Geometry check sheet. Reference: the model listing, model coordinates, mm. Face numbers are marked on the shaded views. A direction names the side the tool comes from. Coordinates: 2 decimals unless noted, no trailing zeros. Loops run counter-clockwise (first coordinate to the right, second up) from the corner with the lowest first, then second, coordinate; pieces in that order, holes last. Notation, with made-up numbers: M 88.5,74 L 118.5,74 A16 cw 118.5,90 Z; hole C -12.75,27 d6. An arc over 180 degrees is marked long. Use CSV: the item, a comma, the result in double quotes.
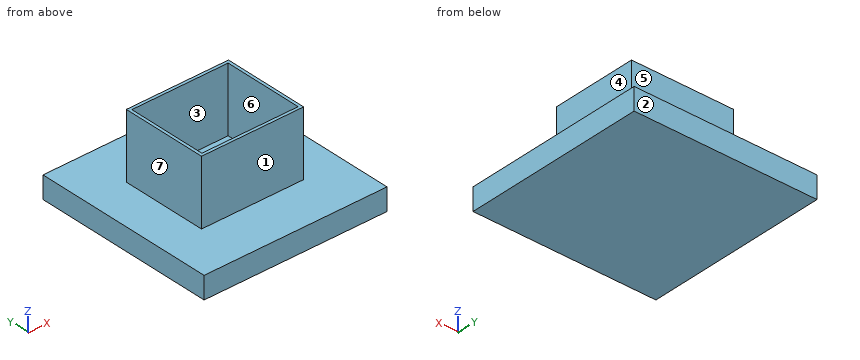
Autodesk Inventor part; units mm, degrees
ref_plane "YZ Plane" through (0, 0, 0) normal (1, 0, 0) x (0, 1, 0)
ref_plane "XZ Plane" through (0, 0, 0) normal (0, 1, 0) x (-1, 0, 0)
ref_plane "XY Plane" through (0, 0, 0) normal (0, 0, 1) x (1, 0, 0)
sketch "Sketch1" plane through (0, 0, 0) normal (0, 0, 1) x (1, 0, 0)
  line L0 (-17.15, -17.15) -> (17.15, -17.15)
  line L1 (17.15, -17.15) -> (17.15, 17.15)
  line L2 (17.15, 17.15) -> (-17.15, 17.15)
  line L3 (-17.15, 17.15) -> (-17.15, -17.15)
  line L4 (-17.15, -17.15) -> (17.15, 17.15) construction
  line L5 (17.15, -17.15) -> (-17.15, 17.15) construction
  point P0 (0, 0)
  dimension "d0" = 34.3
  dimension "d1" = 34.3
extrude "Extrusion1" add sketch "Sketch1" along normal blind 4.15
sketch "Sketch2" plane through (0, 0, 4.15) normal (0, 0, 1) x (1, 0, 0)
  line L0 (-9.025, -7.45) -> (9.025, -7.45)
  line L1 (9.025, -7.45) -> (9.025, 7.45)
  line L2 (9.025, 7.45) -> (-9.025, 7.45)
  line L3 (-9.025, 7.45) -> (-9.025, -7.45)
  line L4 (-9.025, -7.45) -> (9.025, 7.45) construction
  line L5 (9.025, -7.45) -> (-9.025, 7.45) construction
  line L6 (-9.5751, 8.0001) -> (9.5751, 8.0001)
  line L7 (9.5751, 8.0001) -> (9.5751, -8.0001)
  line L8 (9.5751, -8.0001) -> (-9.5751, -8.0001)
  line L9 (-9.5751, -8.0001) -> (-9.5751, 8.0001)
  point P0 (0, 0)
  dimension "d4" = 18.05
  dimension "d5" = 14.9
extrude "Extrusion2" add sketch "Sketch2" along normal blind 12.25
properties part number "RJ45_bulkhead"
1. Section check C-C, the plane x = 3. Record the cut outline in (y, z).
The answers:
outline,"M -17.15,0 L 17.15,0 L 17.15,4.15 L 8,4.15 L 8,16.4 L 7.45,16.4 L 7.45,4.15 L -7.45,4.15 L -7.45,16.4 L -8,16.4 L -8,4.15 L -17.15,4.15 Z"
2. Section check A-A, the plane z = 13.5. Record the cut outline in (x, y) (3 decimals).
The answers:
outline,"M -9.575,-8 L 9.575,-8 L 9.575,8 L -9.575,8 Z; hole M -9.025,-7.45 L 9.025,-7.45 L 9.025,7.45 L -9.025,7.45 Z"
3. Section check B-B, the plane y = -3.5. Record the cut outline in (x, z) (3 decimals), plus the area to 3 significant figures.
The answers:
outline,"M -17.15,0 L 17.15,0 L 17.15,4.15 L 9.575,4.15 L 9.575,16.4 L 9.025,16.4 L 9.025,4.15 L -9.025,4.15 L -9.025,16.4 L -9.575,16.4 L -9.575,4.15 L -17.15,4.15 Z"
area,"156 mm^2"
4. Gauge pin test, flat ends, axial feed: P1, Ø3.5, axis at x = -3, z = 9, coming from the +Y side; P2, Ø3.5, axis at y = -2.5, z = 11, coming from the +X side; P3, Ø1.5, axis at y = 5.5, z = 5, coming from the -X side. Record the tip position at first contact, or that the pin passes through.
The answers:
P1,"y = 8"
P2,"x = 9.58"
P3,"x = -9.58"
5. Section check D-D, the plane y = 14. Record the cut outline in (x, z), plus the area to 3 significant figures.
The answers:
outline,"M -17.15,0 L 17.15,0 L 17.15,4.15 L -17.15,4.15 Z"
area,"142 mm^2"
6. Thickness scan on line 1 (X direction, y = -3, z = 12) (3 decimals); line 2 (Y direction, x = -2, z = 13); line 3 (Z direction, x = -4, y = 14.5). Record the ranges inside material, lowest first. Write a range as [from, to].
The answers:
line 1,"[-9.575, -9.025], [9.025, 9.575]"
line 2,"[-8, -7.45], [7.45, 8]"
line 3,"[0, 4.15]"
7. Set-up check for the marked faces 1, 2 and 3: record each of +Z, -Z, +X, -X, +Y, -Y from which the full face is reachable in a straight line by a thin tool's end or side.
The answers:
face 1,"+Z, +X, -X, -Y"
face 2,"+Z, -Z, +X, -X, +Y"
face 3,"+Z"
8. Release check for a two-part mould opening along X. For the marked faces 4, 5, 6 and 7 record: +X half, -X half, draft (parallel to the pull), parting line (faces both ways), or undercut.
The answers:
face 4,"+X half"
face 5,"draft"
face 6,"undercut"
face 7,"-X half"
